from build123d import *

# Parameters (mm, degrees)
F0_W     = 127
F0_H     = 6.35
F1_DEPTH = 152.4
F3_D     = 4.4958
F4_D     = 13.49248
F5_D     = 4.4958


with BuildPart() as f1:
    # F0 (on Top) → F1 (new body, symmetric)
    with BuildSketch(Plane.XY):
        Rectangle(F0_W, F0_H)
    extrude(amount=F1_DEPTH, both=True)

    # F3 (through all)
    with Locations(Plane(origin=(0, 3.175, 0), x_dir=(-1, 0, 0), z_dir=(0, 1, 0))):
        with Locations((54.7769896194, -124.7698038497), (19.05, -138.0058233698), (-19.05, -138.0058233698), (-54.7769896194, -124.7698038497), (54.7769896194, 61.2698038497), (19.05, 74.5058233698), (-19.05, 74.5058233698), (-54.7769896194, 61.2698038497)):
            Hole(F3_D / 2)

    # F4 (through all)
    with Locations(Plane(origin=(0, 3.175, 0), x_dir=(-1, 0, 0), z_dir=(0, 1, 0))):
        with Locations((0, -31.75)):
            Hole(F4_D / 2)

    # F5 (through all)
    with Locations(Plane(origin=(0, 3.175, 0), x_dir=(-1, 0, 0), z_dir=(0, 1, 0))):
        with Locations((0, -76.2)):
            Hole(F5_D / 2)


solid = f1.part
Part model, mm, in its own coordinate system. Coordinates: 2 decimals unless noted, no trailing zeros. Order: outer loops, then holes, each group sorted by start corner. A loop starts at its lowest first (then second) coordinate and runs counter-clockwise, first axis right, second up. Notation, with made-up numbers: M -14,56.25 L -1,56.25 A8 cw -1,70.25 Z; hole C -20.75,83.5 d7. An arc over 180 degrees is marked long. One line per question, with ' | ' between items.
Q1. Slice it at A-A (z = -31.75). Give the cut face in (x, y) (3 decimals), and give its area (3 significant figures).
A:
outline: M -63.5,-3.175 L -6.746,-3.175 L -6.746,3.175 L -63.5,3.175 Z; M 6.746,-3.175 L 63.5,-3.175 L 63.5,3.175 L 6.746,3.175 Z | area: 721 mm^2
Q2. Drill centre lines: line 1 (Z direction, x = 19.05, y = -1.5); line 2 (Z direction, x = 0, y = 0.5); line 3 (Z direction, x = 2.5, y = -2.5). Where is each one in solid material? Low to high.
A:
line 1: z = -152.4 to -140.25, -135.76 to 72.26, 76.75 to 152.4 | line 2: z = -152.4 to -78.45, -73.95 to -38.5, -25 to 152.4 | line 3: z = -152.4 to -38.02, -25.48 to 152.4
Q3. Two-plate mould, pull along Z, no slides. Class faces 1 (the face through (3.627, -0.044, -26.062)), 2 (the face through (-1, 0, 152.4)), 3 (the face through (-63.5, 0, 2)), 4 (the face through (-1, 0, -152.4)): +Z half, -Z half, draft (parallel to the pull), parting line (faces both ways), or undercut.
A:
face 1: undercut | face 2: +Z half | face 3: draft | face 4: -Z half
